For this review, take the finished solid that the model builds, in its own axes (mm). A direction names the side the tool comes from. Round coordinates to 2 decimals unless told otherwise and drop trailing zeros. Loops run counter-clockwise (first coordinate to the right, second up) from the corner with the lowest first, then second, coordinate; pieces in that order, holes last.
1) Mouldability with a two-part tool opening along Y and no side actions: class faces 5 (the flat face through (9, -11.35, 0)), 6 (the flat face through (10.75, -7.32, -4.97)), 7 (the flat face through (6, -1.5, 4)), 8 (the flat face through (10.72, -7.65, -0.08)) as pulls with the +Y half, pulls with the -Y half, needs draft (parallel to the pull), parting line crosses it, or undercut.
2) Insertion check: pin 1 (10 mm diameter, centred on x = 4, y = -10.5, fed in from +Z); pin 2 (8 mm diameter, centred on y = -14.5, z = 9.5, fed in from -X); pin 3 (4 mm diameter, centred on y = -9.5, z = -8.75, fed in from +X); pin 4 (1.1 mm diameter, centred on x = 5, z = 1.5, fed in from +Y). Each pin has a flat end and moves straight along its axis. Give the tip position at first contact, or say it passes through.
3) Take a section at D-D (y = -14). State the section outline as (x, z) points, then the cut area to 4 significant figures.
4) Take a section at C-C (z = 0). Give the number of separate pieces and of enclosed holes in the cut face, then the cut area to 3 significant figures.
5) Take a section at B-B (x = 7). State the section outline as (y, z) points (3 decimals).
6) Wall thickness on L1, parallel to Z at x = 7, y = -1.6 (3 decimals); L2, parallel to Z at x = 7, y = -0.65; L3, parallel to Y at x = 20.95, z = 8.75: over which ranges is each line inside the solid? List them lowest first.
7) Tool access review of faces 1 (the flat face through (10.476, -7.259, -0.076)), 2 (the cylindrical face through (10.14, -1.72, -12.04)), 3 (the flat face through (9, -11.8, 0)), 4 (the flat face through (20.5, -10, 0)): name each direction out of +Z, -Z, +X, -X, +Y, -Y from which nothing blocks a thin tool from reaching the whole face with its end or side.
8) Take a section at A-A (y = -10.75). State the section outline as (x, z) points.
Autodesk Inventor part; units mm, degrees
ref_plane "side_1_XY" through (22, -9.5, 0) normal (1, 0, 0) x (0, 1, 0)
ref_plane "side_1_YZ" through (22, -9.5, 0) normal (0, 1, 0) x (0, 0, 1)
ref_plane "side_1_ZX" through (22, -9.5, 0) normal (0, 0, 1) x (1, 0, 0)
sketch "Skizze_1" plane through (0, 0, 0) normal (0, 0, 1) x (1, 0, 0)
  line L0 (0, -0.3) -> (0, -1.2)
  arc A0 (0, -1.2) -> (0.3, -1.5) centre (0.3, -1.2) ccw
  line L1 (0.3, -1.5) -> (20.2, -1.5)
  arc A1 (20.5, -1.8) -> (20.2, -1.5) centre (20.2, -1.8) ccw
  line L2 (20.5, -1.8) -> (20.5, -18.7)
  arc A2 (20.5, -18.7) -> (20.8, -19) centre (20.8, -18.7) ccw
  line L3 (20.8, -19) -> (21.7, -19)
  arc A3 (21.7, -19) -> (22, -18.7) centre (21.7, -18.7) ccw
  line L4 (22, -18.7) -> (22, -1)
  arc A4 (22, -1) -> (21, 0) centre (21, -1) ccw
  line L5 (21, 0) -> (0.3, 0)
  arc A5 (0.3, 0) -> (0, -0.3) centre (0.3, -0.3) ccw
extrude "Extrusion1" add sketch "Skizze_1" along normal mid plane 32.5
sketch "Skizze_2" plane through (22, 0, 0) normal (1, 0, 0) x (0, 0, -1)
  circle A0 centre (8.75, -9.5) radius 2.25
extrude "Extrusion2" cut sketch "Skizze_2" along normal mid plane 3
sketch "Skizze_3" plane through (22, 0, 0) normal (1, 0, 0) x (0, 0, -1)
  circle A0 centre (-8.75, -9.5) radius 2.25
extrude "Extrusion3" cut sketch "Skizze_3" along normal mid plane 3
sketch "Skizze_4" plane through (0, 0, 0) normal (0, 0, 1) x (1, 0, 0)
  arc A0 (2.1852, -1.45) -> (0.5463, -5.08) centre (2.1852, -3.635) ccw
  line L0 (0.5463, -5.08) -> (5.946, -10.1545)
  arc A1 (5.4062, -11.35) -> (5.946, -10.1545) centre (5.4062, -10.6304) ccw
  line L1 (5.4062, -11.35) -> (4, -11.35)
  line L2 (4, -11.35) -> (4, -11.8)
  line L3 (4, -11.8) -> (5.3389, -11.8)
  arc A2 (5.3389, -11.8) -> (6.239, -9.8064) centre (5.3389, -10.6) ccw
  line L4 (6.239, -9.8064) -> (0.8838, -4.7824)
  arc A3 (2.1852, -1.9) -> (0.8838, -4.7824) centre (2.1852, -3.635) ccw
  line L5 (2.1852, -1.9) -> (11.8148, -1.9)
  arc A4 (13.1162, -4.7824) -> (11.8148, -1.9) centre (11.8148, -3.635) ccw
  line L6 (13.1162, -4.7824) -> (7.761, -9.8064)
  arc A5 (7.761, -9.8064) -> (8.6611, -11.8) centre (8.6611, -10.6) ccw
  line L7 (8.6611, -11.8) -> (10, -11.8)
  line L8 (10, -11.8) -> (10, -11.35)
  line L9 (10, -11.35) -> (8.5938, -11.35)
  arc A6 (8.054, -10.1545) -> (8.5938, -11.35) centre (8.5938, -10.6304) ccw
  line L10 (8.054, -10.1545) -> (13.4537, -5.08)
  arc A7 (13.4537, -5.08) -> (11.8148, -1.45) centre (11.8148, -3.635) ccw
  line L11 (11.8148, -1.45) -> (2.1852, -1.45)
extrude "Extrusion4" add sketch "Skizze_4" along normal mid plane 12
sketch "Skizze_5" plane through (0, 0, 0) normal (0, 1, 0) x (-1, 0, 0)
  line L0 (-1.809, 5.7484) -> (-2.5923, 9.8744)
  arc A0 (-2.5923, 9.8744) -> (-6.2765, 12.925) centre (-6.2765, 9.175) ccw
  line L1 (-6.2765, 12.925) -> (-7.7235, 12.925)
  arc A1 (-7.7235, 12.925) -> (-11.4077, 9.8744) centre (-7.7235, 9.175) ccw
  line L2 (-11.4077, 9.8744) -> (-12.191, 5.7484)
  line L3 (-12.191, 5.7484) -> (-12.191, -5.7484)
  line L4 (-12.191, -5.7484) -> (-11.4077, -9.8744)
  arc A2 (-11.4077, -9.8744) -> (-7.7235, -12.925) centre (-7.7235, -9.175) ccw
  line L5 (-7.7235, -12.925) -> (-6.2765, -12.925)
  arc A3 (-6.2765, -12.925) -> (-2.5923, -9.8744) centre (-6.2765, -9.175) ccw
  line L6 (-2.5923, -9.8744) -> (-1.809, -5.7484)
  line L7 (-1.809, -5.7484) -> (-1.809, 5.7484)
extrude "Extrusion5" add sketch "Skizze_5" against normal blind 1.94
sketch "Skizze_6_ALT_Drilling_1" plane through (0, 0, 0) normal (0, 1, 0) x (-1, 0, 0)
  circle A0 centre (-7, 0) radius 5.5
extrude "Extrusion6" cut sketch "Skizze_6_ALT_Drilling_1" against normal blind 1.5
sketch "Skizze_7_ALT_Drilling_2" plane through (0, 0, 0) normal (0, 1, 0) x (-1, 0, 0)
  circle A0 centre (-7, 0) radius 3.825
extrude "Extrusion7" cut sketch "Skizze_7_ALT_Drilling_2" against normal blind 2.6
sketch "Skizze_8" plane through (17, 0, 0) normal (1, 0, 0) x (0, 0, -1)
  line L0 (-6, -1.94) -> (-6, -12.9)
  line L1 (-6, -12.9) -> (-3.9, -12.9)
  line L2 (-3.9, -12.9) -> (-6, -1.94)
extrude "Extrusion8" cut sketch "Skizze_8" against normal blind 30
sketch "Skizze_9" plane through (17, 0, 0) normal (1, 0, 0) x (0, 0, -1)
  line L0 (3.9, -12.9) -> (6, -12.9)
  line L1 (6, -12.9) -> (6, -1.94)
  line L2 (6, -1.94) -> (3.9, -12.9)
extrude "Extrusion9" cut sketch "Skizze_9" against normal blind 30
sketch "Skizze_10_ALT_Drilling_3" plane through (0, 0, 0) normal (0, 1, 0) x (-1, 0, 0)
  circle A0 centre (-7, 9) radius 0.75
extrude "Extrusion10" cut sketch "Skizze_10_ALT_Drilling_3" against normal blind 3
sketch "Skizze_11_ALT_Drilling_4" plane through (0, 0, 0) normal (0, 1, 0) x (-1, 0, 0)
  circle A0 centre (-7, -9) radius 0.75
extrude "Extrusion11" cut sketch "Skizze_11_ALT_Drilling_4" against normal blind 3
sketch "Skizze_12" plane through (0, -11.8, 0) normal (0, 1, 0) x (1, 0, 0)
  line L0 (3, -5.05) -> (11, -5.05)
  line L1 (11, -5.05) -> (11, 5.05)
  line L2 (11, 5.05) -> (3, 5.05)
  line L3 (3, 5.05) -> (3, -5.05)
  arc A0 (4, -2.55) -> (5.5, -4.05) centre (5.5, -2.55) ccw
  line L4 (5.5, -4.05) -> (8.5, -4.05)
  arc A1 (8.5, -4.05) -> (10, -2.55) centre (8.5, -2.55) ccw
  line L5 (10, -2.55) -> (10, 2.55)
  arc A2 (10, 2.55) -> (8.5, 4.05) centre (8.5, 2.55) ccw
  line L6 (8.5, 4.05) -> (5.5, 4.05)
  arc A3 (5.5, 4.05) -> (4, 2.55) centre (5.5, 2.55) ccw
  line L7 (4, 2.55) -> (4, -2.55)
extrude "Extrusion12" cut sketch "Skizze_12" along normal blind 0.45
ref_plane "side_1_XY" through (22, -9.5, 0) normal (1, 0, 0) x (0, 1, 0)
ref_plane "side_1_YZ" through (22, -9.5, 0) normal (0, 1, 0) x (0, 0, 1)
ref_plane "side_1_ZX" through (22, -9.5, 0) normal (0, 0, 1) x (1, 0, 0)
ref_plane "side_2_XY" through (7, -1.6, 0) normal (0, 1, 0) x (1, 0, 0)
ref_plane "side_2_YZ" through (7, -1.6, 0) normal (1, 0, 0) x (0, 0, -1)
ref_plane "side_2_ZX" through (7, -1.6, 0) normal (0, 0, -1) x (0, 1, 0)
properties part number "May Tec 1.64.5101._Mounting angle"
Response:
1. face 5: undercut
1. face 6: pulls with the -Y half
1. face 7: pulls with the +Y half
1. face 8: undercut
2. pin 1: stops at z = 5.24
2. pin 2: stops at x = 20.5
2. pin 3: passes through
2. pin 4: stops at y = -8.13
3. outline: (20.5, -16.25) - (22, -16.25) - (22, 16.25) - (20.5, 16.25) - close
3. area: 48.75 mm2
4. separate pieces: 4
4. enclosed holes: 0
4. area: 57.1 mm2
5. outline: (-1.94, -12.925) - (-1.5, -12.925) - (-1.5, -16.25) - (0, -16.25) - (0, -9.75) - (-1.94, -9.75) - close; (-1.94, -8.25) - (0, -8.25) - (0, -5.5) - (-1.5, -5.5) - (-1.5, -3.825) - (-1.94, -3.825) - close; (-1.94, 3.825) - (-1.5, 3.825) - (-1.5, 5.5) - (0, 5.5) - (0, 8.25) - (-1.94, 8.25) - close; (-1.94, 9.75) - (0, 9.75) - (0, 16.25) - (-1.5, 16.25) - (-1.5, 12.925) - (-1.94, 12.925) - close
6. L1: z = -12.925 to -9.75, -8.25 to -3.825, 3.825 to 8.25, 9.75 to 12.925
6. L2: z = -16.25 to -9.75, -8.25 to -5.5, 5.5 to 8.25, 9.75 to 16.25
6. L3: y = -19 to -11.75, -7.25 to 0
7. face 1: +Z, -Z
7. face 2: -Z, -Y
7. face 3: +Z, -Z, -X, -Y
7. face 4: +Z, -Z, -Y
8. outline: (6.12, -4.31) - (6.53, -4.31) - (6.53, 4.31) - (6.12, 4.31) - close; (7.47, -4.31) - (7.88, -4.31) - (7.88, 4.31) - (7.47, 4.31) - close; (20.5, -16.25) - (22, -16.25) - (22, -10.62) - (20.5, -10.62) - close; (20.5, -6.88) - (22, -6.88) - (22, 6.88) - (20.5, 6.88) - close; (20.5, 10.62) - (22, 10.62) - (22, 16.25) - (20.5, 16.25) - close
